```python
from build123d import *

# Parameters (mm, degrees)
CUT_EXTRUDE_1_DEPTH = 1
SKETCH_3_R          = 1
EXTRUDE_2_DEPTH     = 8


with BuildPart() as part:
    # 草图1 → 旋转1 (revolve)
    with BuildSketch(Plane.XY):
        Polygon((0, -1.2), (0, 0), (1.8, 0), (1.8, -0.1), (1, -1.2), align=None)
    revolve(axis=Axis((0, 0, 0), (0, 1, 0)))

    # 草图2 → 切除-拉伸1 (cut)
    with BuildSketch(Plane(origin=(0, 0, 0), x_dir=(1, 0, 0), z_dir=(0, 1, 0))):
        Polygon((0, -0.866025404), (0.75, -0.433012702), (0.75, 0.433012702), (0, 0.866025404), (-0.75, 0.433012702), (-0.75, -0.433012702), align=None)
    extrude(amount=-CUT_EXTRUDE_1_DEPTH, mode=Mode.SUBTRACT)

    # 草图3 → 凸台-拉伸2 (add)
    with BuildSketch(Plane.XZ.offset(1.2)):
        Circle(SKETCH_3_R)
    extrude(amount=EXTRUDE_2_DEPTH)


solid = part.part
```
Input: part model. Units: mm. Frame: model coordinates. A direction names the side the tool comes from. Coordinates: 2 decimals unless noted, no trailing zeros. Loops run counter-clockwise (first coordinate to the right, second up) from the corner with the lowest first, then second, coordinate; pieces in that order, holes last.
Q1. Line query: line 1 along Y through (x, z) = (0.7, -0.3); line 2 along Z through (x, y) = (0.9, -8); line 3 along X through (y, z) = (-5.25, -0.5). Output: solid intervals per line, ascending.
Results are:
line 1: y = -9.2 to -1
line 2: z = -0.44 to 0.44
line 3: x = -0.87 to 0.87
Q2. Set-up query: faces 1 (the flat face through (-1, 0, 0)), 2 (the flat face through (0, -1, 0)), 3 (the cylindrical face through (0, -5, -1)). Return all of +Z, -Z, +X, -X, +Y, -Y with unobstructed straight access to the full face (end or side cutting, diameter ignored); none if empty.
Results are:
face 1: +Z, -Z, +X, -X, +Y
face 2: +Y
face 3: -Y
Q3. Section A-A, the plane z = 0. Return the cut outline in (x, y).
Results are:
outline: (-1.8, -0.1) - (-1, -1.2) - (-1, -9.2) - (1, -9.2) - (1, -1.2) - (1.8, -0.1) - (1.8, 0) - (0.75, 0) - (0.75, -1) - (-0.75, -1) - (-0.75, 0) - (-1.8, 0) - close
Q4. Contact query for flat-ended pins moving along their axis: pin 1 (1.5 mm diameter, centred on y = -3, z = 0.5, fed in from +X); pin 2 (2 mm diameter, centred on x = 0.5, y = -3, fed in from -Z); pin 3 (0.7 mm diameter, centred on y = -0.5, z = 0, fed in from +X). Output: stop coordinate, or through.
Results are:
pin 1: stops at x = 1
pin 2: stops at z = -1
pin 3: stops at x = 1.76
Q5. Section B-B, the plane y = -0.75. Return the cut outline in (x, z), and give its area (3 significant figures).
Results are:
outline: circle Ø2.65 at (0, 0); hole (-0.75, -0.43) - (0, -0.87) - (0.75, -0.43) - (0.75, 0.43) - (0, 0.87) - (-0.75, 0.43) - close
area: 3.59 mm2
Q6. Section C-C, the plane y = -3.25. Return the cut outline in (x, z), and give its area (3 significant figures).
Results are:
outline: circle Ø2 at (0, 0)
area: 3.14 mm2
